The listing builds one solid part. Answer for the finished solid, in the listing's coordinates (mm). A direction names the side the tool comes from. Give positions to 0.01 mm unless a question says otherwise; leave off trailing zeros. Loops run counter-clockwise (first coordinate to the right, second up) from the corner with the lowest first, then second, coordinate; pieces in that order, holes last.
Item 1: Section D-D, the plane y = -18 is taken. Give the vertices of the cut face in (x, z).
Item 2: Section A-A, the plane x = 0 is taken. Give the number of separate pieces and of enclosed holes in the cut face, and give its area (3 significant figures).
Item 3: A tool of negligible diameter and unlimited length cuts with its end or side. For faces 1 (the face through (-3.48, -1.97, 5.46)), 2 (the face through (10, -20, 0)), 3 (the face through (-20, 10, 0)), from which of +Z, -Z, +X, -X, +Y, -Y can it reach the whole face along a straight path? Write none if from no direction.
Item 4: Each of these flat-tipped pins is pushed along its axis until it touches: pin 1 Ø3.5 at (x, y) = (25, 0) entering from -Z; pin 2 Ø5 at (x, z) = (-1, 6) entering from -Y; pin 3 Ø1.5 at (x, z) = (-23, -0.5) entering from +Y; pin 4 Ø5 at (x, y) = (21.5, 6) entering from +Z. Where does it stop, or does it pass through?
Item 5: Section B-B, the plane z = 4.5 is taken. Give the vertices of the cut face in (x, y), and give its area (3 significant figures).
Item 6: Section C-C, the plane z = -1.25 is taken. Give the vertices of the cut face in (x, y), and give its area (3 significant figures).
Item 7: The mould has two halves that part along Y. Classify faces 4 (the face through (-7.493, 0.33, 5.458)), 5 (the face through (-0.1, 27.9, 0.2)), 6 (the face through (20, -10, 0)): pulls with the +Y half, pulls with the -Y half, needs draft (parallel to the pull), parting line crosses it, or undercut.
Item 8: Consider line 1 along X through (y, z) = (0, -1.3); line 2 along Y through (x, z) = (0, -0.6); line 3 along X through (y, z) = (0, -1.8). Determine where each line is inside the solid, lowest interval first.
from build123d import *

# Parameters (mm, degrees)
EXTRUDE_1_DEPTH             = 2.5
HOLE_WIZARD_M5_1_AT_2_COUNT = 2
HOLE_WIZARD_M5_1_AT_2_PITCH = 50
HOLE_WIZARD_M5_1_AT_3_COUNT = 2
HOLE_WIZARD_M5_1_AT_3_PITCH = 35.355339059
HOLE_WIZARD_M5_1_AT_4_COUNT = 2
HOLE_WIZARD_M5_1_AT_4_PITCH = 35.355339059
FILLET_1_R                  = 5
SKETCH_14_R                 = 7.5
EXTRUDE_2_DEPTH             = 6


with BuildPart() as part:
    # 草圖1 → 填料-伸長1 (new, symmetric)
    with BuildSketch(Plane.XY):
        with BuildLine():
            Line((10, 25), (10, 10))
            Line((10, 10), (25, 10))
            ThreePointArc((25, 10), (35, 0), (25, -10))
            Line((25, -10), (10, -10))
            Line((10, -10), (10, -25))
            ThreePointArc((10, -25), (0, -35), (-10, -25))
            Line((-10, -25), (-10, -10))
            Line((-10, -10), (-25, -10))
            ThreePointArc((-25, -10), (-35, 0), (-25, 10))
            Line((-25, 10), (-10, 10))
            Line((-10, 10), (-10, 25))
            ThreePointArc((-10, 25), (0, 35), (10, 25))
        make_face()
    extrude(amount=EXTRUDE_1_DEPTH, both=True)

    # 草圖6 → M5 錐坑平頭螺釘的錐孔1 (revolve, cut)
    with BuildSketch(Plane(origin=(0, 25, 2.5), x_dir=(0, -1, 0), z_dir=(1, 0, 0))):
        Polygon((0, 0), (0, 5), (2.75, 5), (2.75, 2.45), (5.2, 0), align=None)
    hole_wizard_m5_1 = revolve(axis=Axis((0, 25, 8.85), (0, 0, -1)), mode=Mode.SUBTRACT)

    # M5 錐坑平頭螺釘的錐孔1 at 2: M5 錐坑平頭螺釘的錐孔1 ×2
    with Locations(*[(0, -i * HOLE_WIZARD_M5_1_AT_2_PITCH, 0) for i in range(1, HOLE_WIZARD_M5_1_AT_2_COUNT)]):
        add(hole_wizard_m5_1, mode=Mode.SUBTRACT)

    # M5 錐坑平頭螺釘的錐孔1 at 3: M5 錐坑平頭螺釘的錐孔1 ×2
    with Locations(*[Vector(0.7071067811865479, -0.7071067811865472, 0) * (i * HOLE_WIZARD_M5_1_AT_3_PITCH) for i in range(1, HOLE_WIZARD_M5_1_AT_3_COUNT)]):
        add(hole_wizard_m5_1, mode=Mode.SUBTRACT)

    # M5 錐坑平頭螺釘的錐孔1 at 4: M5 錐坑平頭螺釘的錐孔1 ×2
    with Locations(*[Vector(-0.7071067811865476, -0.7071067811865476, 0) * (i * HOLE_WIZARD_M5_1_AT_4_PITCH) for i in range(1, HOLE_WIZARD_M5_1_AT_4_COUNT)]):
        add(hole_wizard_m5_1, mode=Mode.SUBTRACT)

    # 圓角1
    fillet_1_edges = [part.edges().sort_by_distance(p)[0] for p in [
        (10, 10, 0),
        (10, -10, 0),
        (-10, -10, 0),
        (-10, 10, 0),
    ]]
    fillet(fillet_1_edges, radius=FILLET_1_R)

    # 草圖13 → M5 錐坑平頭螺釘的錐孔3 (revolve, cut)
    with BuildSketch(Plane(origin=(0, 0, -2.5), x_dir=(0, 1, 0), z_dir=(1, 0, 0))):
        Polygon((0, 0), (0, 5), (2.75, 5), (2.75, 2.45), (5.2, 0), align=None)
    revolve(axis=Axis((0, 0, -8.85), (0, 0, 1)), mode=Mode.SUBTRACT)

    # 草圖14 → 填料-伸長2 (add)
    with BuildSketch(Plane.XY.offset(2.5)):
        Circle(SKETCH_14_R)
        Polygon((2.309401077, 4), (-2.309401077, 4), (-4.618802154, 0), (-2.309401077, -4), (2.309401077, -4), (4.618802154, 0), align=None, mode=Mode.SUBTRACT)
    extrude(amount=EXTRUDE_2_DEPTH)


solid = part.part
Worked answers:
1. outline: (-10, -2.5) - (10, -2.5) - (10, 2.5) - (-10, 2.5) - close
2. separate pieces: 4
2. enclosed holes: 0
2. area: 291 mm2
3. face 1: +Z
3. face 2: +Z, -Z, +X, -Y
3. face 3: +Z, -Z, -X, +Y
4. pin 1: passes through
4. pin 2: stops at y = -7.5
4. pin 3: stops at y = 10
4. pin 4: stops at z = 2.5
5. outline: circle Ø15 at (0, 0); hole (-4.62, 0) - (-2.31, -4) - (2.31, -4) - (4.62, 0) - (2.31, 4) - (-2.31, 4) - close
5. area: 121 mm2
6. outline: (-25, -10) - (-15, -10) arc R5 cw to (-10, -15) - (-10, -25) arc R10 ccw to (10, -25) - (10, -15) arc R5 cw to (15, -10) - (25, -10) arc R10 ccw to (25, 10) - (15, 10) arc R5 cw to (10, 15) - (10, 25) arc R10 ccw to (-10, 25) - (-10, 15) arc R5 cw to (-15, 10) - (-25, 10) arc R10 ccw to start; hole circle Ø5.5 at (-25, 0); hole circle Ø7.9 at (0, 0); hole circle Ø5.5 at (0, -25); hole circle Ø5.5 at (0, 25); hole circle Ø5.5 at (25, 0)
6. area: 2,110 mm2
7. face 4: parting line crosses it
7. face 5: undercut
7. face 6: pulls with the -Y half
8. line 1: x = -35 to -27.75, -22.25 to -4, 4 to 22.25, 27.75 to 35
8. line 2: y = -35 to -27.75, -22.25 to -3.3, 3.3 to 22.25, 27.75 to 35
8. line 3: x = -35 to -27.75, -22.25 to -4.5, 4.5 to 22.25, 27.75 to 35
